Here's how the part is built. I have some questions about the finished solid (model axes, mm). A direction names the side the tool comes from. Coordinates: 2 decimals unless noted, no trailing zeros. Write each loop counter-clockwise with the first axis right and the second up, starting at its lowest first coordinate (ties: lowest second). Pieces come first, ordered by that corner, then holes.
Item 1: I'm going to push flat-ended pins straight in: pin 1 Ø1 at (x, y) = (0.5, -0.5) entering from -Z; pin 2 Ø1.5 at (x, z) = (1, -1.5) entering from -Y; pin 3 Ø1 at (y, z) = (1.5, 1) entering from -X. Where does each tip first touch, or does it pass through?
Item 2: For faces 1 (the face through (-0.434, -1.952, -2.254)), 2 (the face through (-0.434, -1.952, 2.246)), which set-ups out of +Z, -Z, +X, -X, +Y, -Y let a thin tool reach every point of the face, with its end or its side?
Item 3: We'd pull the mould along Y, two halves only. Please class faces 3 (the face through (-0.5, 0, -2)), 4 (the face through (-0.29, 2.23, 0.03)): +Y half, -Y half, draft (parallel to the pull), parting line (faces both ways), or undercut.
Item 4: If we section it at B-B (x = -0.2): Count the separate pieces of the cut face and the enclosed holes in it, then the cut area to 3 significant figures.
Item 5: If I drill on line 1 (Y direction, x = 0.15, z = -1.7) (3 decimals); line 2 (Y direction, x = 0.75, z = 1.55); line 3 (X direction, y = 0.45, z = 1.3), over which ranges is the centre line in solid material (lowest first)?
Item 6: If we section it at A-A (z = 0.45): Please give me the cut outline in (x, y), then the cut area to 3 significant figures.
from build123d import *

# Parameters (mm, degrees)
F0_R     = 2
F0_R_2   = 0.284
F1_DEPTH = 2
F0_R_3   = 2.25
F2_DEPTH = 2.5
F4_DEPTH = 12.5


# Not quite as in the source:
# - a fillet or chamfer that OpenCascade refuses, or shapes differently, is made with other operations: its cross-section is extruded or revolved along the edge and cut away or added


with BuildPart() as f1:
    # F0 (on Top) → F1 (new body, symmetric)
    with BuildSketch(Plane.XY):
        Circle(F0_R)
        Circle(F0_R_2, mode=Mode.SUBTRACT)
    extrude(amount=F1_DEPTH, both=True)

    # F0 (on Top) → F2 (join, symmetric)
    with BuildSketch(Plane.XY):
        Circle(F0_R_3)
        Circle(F0_R, mode=Mode.SUBTRACT)
    extrude(amount=F2_DEPTH, both=True)

    # F3 (on Top) → F4 (cut, symmetric)
    with BuildSketch(Plane.XY):
        Polygon((0.4010943762, 1.1171780688), (0, 1.7317327438), (-0.4010943762, 1.1171780688), (0, 0.5784067907), align=None)
        Polygon((-0.8970670571, 0.7371121703), (-1.605488264, 0.5455565888), (-1.1449570143, -0.0258146699), (-0.508610101, 0.1891592692), align=None)
        Polygon((-0.9367568521, -0.6149595416), (-0.9734908601, -1.3479020768), (-0.2877725187, -1.0864742598), (-0.2955828739, -0.4148417807), align=None)
        Polygon((0.3368749389, -1.0705199164), (1.0225932803, -1.3319477334), (0.9858592722, -0.5990051982), (0.344685294, -0.3988874373), align=None)
        Polygon((1.1637124699, 0), (1.6242437196, 0.5713712587), (0.9158225127, 0.7629268403), (0.5273655565, 0.2149739391), align=None)
    extrude(amount=F4_DEPTH, both=True, mode=Mode.SUBTRACT)

    # F5: fillet of radius 0.3 on 3 edges, made by hand

    # F5_s1 → F5_t2 (revolve, cut)
    with BuildSketch(Plane.XZ):
        with BuildLine():
            ThreePointArc((2.25, -2.2041960108), (2.1791287847, -2.3978451782), (2, -2.5))
            Line((2, -2.5), (2.25, -2.5))
            Line((2.25, -2.5), (2.25, -2.2041960108))
        make_face()
    revolve(axis=Axis((0, 0, -2.5), (0, 0, 1)), mode=Mode.SUBTRACT)

    # F5_s3 → F5_t4 (revolve, cut)
    with BuildSketch(Plane.XZ):
        with BuildLine():
            ThreePointArc((2.25, 2.2041960108), (2.1791287847, 2.3978451782), (2, 2.5))
            Line((2, 2.5), (2.25, 2.5))
            Line((2.25, 2.5), (2.25, 2.2041960108))
        make_face()
    revolve(axis=Axis((0, 0, 2.5), (0, 0, 1)), mode=Mode.SUBTRACT)


solid = f1.part
Answer list:
1. pin 1: stops at z = -2
1. pin 2: stops at y = -2.24
1. pin 3: stops at x = -2.02
2. face 1: -Z
2. face 2: +Z
3. face 3: undercut
3. face 4: parting line
4. separate pieces: 3
4. enclosed holes: 0
4. area: 14.4 mm2
5. line 1: y = -2.245 to -0.241, 0.241 to 0.78, 1.502 to 2.245
5. line 2: y = -2.12 to -1.23, -0.53 to 0.14, 0.53 to 2.12
5. line 3: x = -2.2 to -1.53, -0.69 to 0.69, 1.53 to 2.2
6. outline: circle Ø4.5 at (0, 0); hole (-1.61, 0.55) - (-1.14, -0.03) - (-0.51, 0.19) - (-0.9, 0.74) - close; hole (-0.97, -1.35) - (-0.29, -1.09) - (-0.3, -0.41) - (-0.94, -0.61) - close; hole (-0.4, 1.12) - (0, 0.58) - (0.4, 1.12) - (0, 1.73) - close; hole circle Ø0.57 at (0, 0); hole (0.34, -1.07) - (1.02, -1.33) - (0.99, -0.6) - (0.34, -0.4) - close; hole (0.53, 0.21) - (1.16, 0) - (1.62, 0.57) - (0.92, 0.76) - close
6. area: 13.3 mm2
